```python
from build123d import *

# Parameters (mm, degrees)
SKETCH1_R           = 8
SKETCH1_R_2         = 2.5
BOSS_EXTRUDE1_DEPTH = 5
SKETCH2_R           = 6.8
SKETCH2_R_2         = 4.15
CUT_EXTRUDE1_DEPTH  = 0.1
SKETCH3_R           = 6.8
SKETCH3_R_2         = 4.15
CUT_EXTRUDE2_DEPTH  = 0.1


with BuildPart() as part:
    # Sketch1 → Boss-Extrude1 (new body)
    with BuildSketch(Plane(origin=(0, 0, 0), x_dir=(1, 0, 0), z_dir=(0, 1, 0))):
        Circle(SKETCH1_R)
        Circle(SKETCH1_R_2, mode=Mode.SUBTRACT)
    extrude(amount=BOSS_EXTRUDE1_DEPTH)

    # Sketch2 → Cut-Extrude1 (cut)
    with BuildSketch(Plane(origin=(0, 5, 0), x_dir=(1, 0, 0), z_dir=(0, 1, 0))):
        Circle(SKETCH2_R)
        Circle(SKETCH2_R_2, mode=Mode.SUBTRACT)
    extrude(amount=-CUT_EXTRUDE1_DEPTH, mode=Mode.SUBTRACT)

    # Sketch3 → Cut-Extrude2 (cut)
    with BuildSketch(Plane.XZ):
        Circle(SKETCH3_R)
        Circle(SKETCH3_R_2, mode=Mode.SUBTRACT)
    extrude(amount=-CUT_EXTRUDE2_DEPTH, mode=Mode.SUBTRACT)


solid = part.part
```
Part model, mm, in its own coordinate system. A direction names the side the tool comes from. Give positions to 0.01 mm unless a question says otherwise; leave off trailing zeros. Loops run counter-clockwise (first coordinate to the right, second up) from the corner with the lowest first, then second, coordinate; pieces in that order, holes last. Notation, with made-up numbers: M -6,-40 L 0,-40 A22 cw 0,-29 Z; hole C 34,19 d6. An arc over 180 degrees is marked long. Return JSON: item names as keys, results as strings.
1) Saw through at B-B, the plane z = 2. List the corners of the cut face in (x, y).
Calculated:
{"outline": "M -7.75,0 L -6.5,0 L -6.5,0.1 L -3.64,0.1 L -3.64,0 L -1.5,0 L -1.5,5 L -3.64,5 L -3.64,4.9 L -6.5,4.9 L -6.5,5 L -7.75,5 Z; M 1.5,0 L 3.64,0 L 3.64,0.1 L 6.5,0.1 L 6.5,0 L 7.75,0 L 7.75,5 L 6.5,5 L 6.5,4.9 L 3.64,4.9 L 3.64,5 L 1.5,5 Z"}
2) Drill centre lines: line 1 (Z direction, x = 0, y = 0.05); line 2 (X direction, y = 0.15, z = 0); line 3 (Y direction, x = -2.75, z = 4). Where is each one in solid material? Low to high.
Calculated:
{"line 1": "z = -8 to -6.8, -4.15 to -2.5, 2.5 to 4.15, 6.8 to 8", "line 2": "x = -8 to -2.5, 2.5 to 8", "line 3": "y = 0.1 to 4.9"}
3) Flat gauge pins, fed straight in: pin 1 Ø4 at (x, z) = (0, 0) entering from +Y; pin 2 Ø1 at (x, z) = (-4, 2.5) entering from -Y; pin 3 Ø2 at (x, y) = (2, 3) entering from -Z; pin 4 Ø3 at (y, z) = (3, -3.5) entering from -X. Where does each tip first touch, or does it go through?
Calculated:
{"pin 1": "passes through", "pin 2": "stops at y = 0.1", "pin 3": "stops at z = -7.94", "pin 4": "stops at x = -7.75"}
4) Saw through at C-C, the plane y = 4.35. List the corners of the cut face in (x, z), then the cut area to 3 significant figures.
Calculated:
{"outline": "C 0,0 d16; hole C 0,0 d5", "area": "181 mm2"}
5) Saw through at A-A, the plane x = 0. List the corners of the cut face in (y, z).
Calculated:
{"outline": "M 0,-8 L 5,-8 L 5,-6.8 L 4.9,-6.8 L 4.9,-4.15 L 5,-4.15 L 5,-2.5 L 0,-2.5 L 0,-4.15 L 0.1,-4.15 L 0.1,-6.8 L 0,-6.8 Z; M 0,2.5 L 5,2.5 L 5,4.15 L 4.9,4.15 L 4.9,6.8 L 5,6.8 L 5,8 L 0,8 L 0,6.8 L 0.1,6.8 L 0.1,4.15 L 0,4.15 Z"}
6) Pull direction Z, two halves, no side cores. Call faces 4 (the face through (-0.54, 2.46, 2.44)), 5 (the face through (2, 5, 2)), 6 (the face through (-1.73, 2.46, 7.81)): released by +Z, released by -Z, zero draft, split by the parting line, or undercut.
Calculated:
{"face 4": "undercut", "face 5": "zero draft", "face 6": "split by the parting line"}
7) 3-axis set-ups, long thin cutter, end or side, ignore diameter. For faces 1 (the face through (-0.1, 4.9, 4.4)), 2 (the face through (2, 0, 2)), 3 (the face through (-0.1, 0.1, -4.4)): which of +Z, -Z, +X, -X, +Y, -Y reach the whole face in a straight line?
Calculated:
{"face 1": "+Y", "face 2": "+Z, -Z, +X, -X, -Y", "face 3": "-Y"}
8) Saw through at D-D, the plane x = -5.5. List the corners of the cut face in (y, z).
Calculated:
{"outline": "M 0,-5.81 L 5,-5.81 L 5,-4 L 4.9,-4 L 4.9,4 L 5,4 L 5,5.81 L 0,5.81 L 0,4 L 0.1,4 L 0.1,-4 L 0,-4 Z"}
